The listing builds one solid part. Answer for the finished solid, in the listing's coordinates (mm). Face numbers are marked on the shaded views. Coordinates: 2 decimals unless noted, no trailing zeros. Loops run counter-clockwise (first coordinate to the right, second up) from the corner with the lowest first, then second, coordinate; pieces in that order, holes last. Notation, with made-up numbers: (5.5, 69.25) - (49.5, 69.25) arc R31 cw to (49.5, 94.25) - close; hole circle Ø8 at (22, 75.5). An arc over 180 degrees is marked (long way). Return JSON: item names as keys, results as strings. Group by question number.
1. Find the intervals of material crossed by line 1 along Y through (x, z) = (-659, -26.5); line 2 along Z through (x, y) = (303, -25.5); line 3 along Y through (x, z) = (-321.5, 32), in increasing order.
2. The mould has two halves that part along Z. Classify the marked faces 1, 2 and 3: pulls with the +Z half, pulls with the -Z half, needs draft (parallel to the pull), parting line crosses it, or undercut.
3. Section C-C (y = -14) is taken. Write down the section's boundary in (x, z).
4. Section B-B (z = 17.5) is taken. Write down the section's boundary in (x, y), and give its area (3 significant figures).
5. Section A-A (x = -591) is taken. Write down the section's boundary in (y, z), and give its area (3 significant figures).
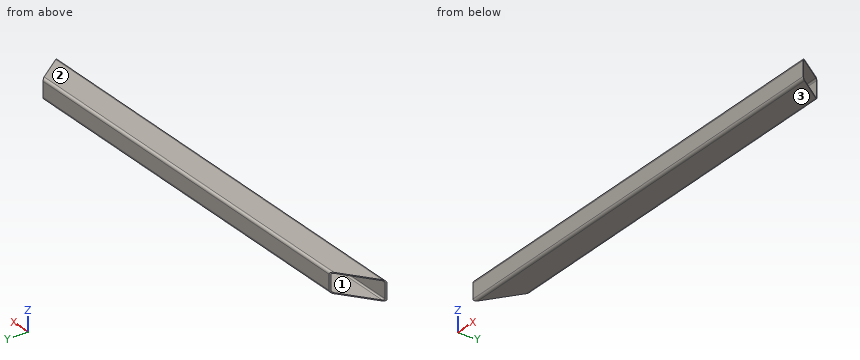
```python
from build123d import *

# Parameters (mm, degrees)
EL_MENT_M_CANO_SOUD_1_DEPTH = 1883.6164
EXTRUSION1_DEPTH            = 81
EXTRUSION2_DEPTH            = 81


with BuildPart() as part:
    # Esquisse15 → Elément mécano-soudé1 (new body)
    with BuildSketch(Plane.YZ.offset(-941.8082)):
        with BuildLine():
            Line((-50, 40), (50, 40))
            ThreePointArc((50, 40), (57.071067812, 37.071067812), (60, 30))
            Line((60, 30), (60, -30))
            ThreePointArc((60, -30), (57.071067812, -37.071067812), (50, -40))
            Line((50, -40), (-50, -40))
            ThreePointArc((-50, -40), (-57.071067812, -37.071067812), (-60, -30))
            Line((-60, -30), (-60, 30))
            ThreePointArc((-60, 30), (-57.071067812, 37.071067812), (-50, 40))
        make_face()
        with BuildLine():
            Line((-50, 36), (50, 36))
            ThreePointArc((50, 36), (54.242640687, 34.242640687), (56, 30))
            Line((56, 30), (56, -30))
            ThreePointArc((56, -30), (54.242640687, -34.242640687), (50, -36))
            Line((50, -36), (-50, -36))
            ThreePointArc((-50, -36), (-54.242640687, -34.242640687), (-56, -30))
            Line((-56, -30), (-56, 30))
            ThreePointArc((-56, 30), (-54.242640687, 34.242640687), (-50, 36))
        make_face(mode=Mode.SUBTRACT)
    extrude(amount=EL_MENT_M_CANO_SOUD_1_DEPTH)

    # Esquisse12 → Extrusion1 (cut, through all)
    with BuildSketch(Plane.XY.offset(40)):
        Polygon((941.8082, -60), (851.381713988, 60), (941.8082, 60), align=None)
        Polygon((-941.8082, -60), (-782.562821406, 60), (-941.8082, 60), align=None)
    extrude(amount=-EXTRUSION1_DEPTH, mode=Mode.SUBTRACT)

    # Esquisse13 → Extrusion2 (cut, through all)
    with BuildSketch(Plane.XY.offset(40)):
        Polygon((-1042.175315796, -60), (-925.191798589, -60), (-765.946419994, 60), (-882.929937201, 60), align=None)
    extrude(amount=-EXTRUSION2_DEPTH, mode=Mode.SUBTRACT)


solid = part.part
```
The answers:
{
 "1": {"line 1": "y = -60 to -56, 56 to 60", "line 2": "z = -40 to -36, 36 to 40", "line 3": "y = -59.8 to -55.66, 55.66 to 59.8"},
 "2": {"face 1": "undercut", "face 2": "pulls with the +Z half", "face 3": "pulls with the -Z half"},
 "3": {"outline": "(-864.15, -40) - (907.14, -40) - (907.14, -36) - (-864.15, -36) - close; (-864.15, 36) - (907.14, 36) - (907.14, 40) - (-864.15, 40) - close"},
 "4": {"outline": "(-925.19, -60) - (941.81, -60) - (938.79, -56) - (-919.88, -56) - close; (-771.25, 56) - (854.4, 56) - (851.38, 60) - (-765.95, 60) - close", "area": "13,900 mm2"},
 "5": {"outline": "(-60, -30) arc R10 ccw to (-50, -40) - (50, -40) arc R10 ccw to (60, -30) - (60, 30) arc R10 ccw to (50, 40) - (-50, 40) arc R10 ccw to (-60, 30) - close; hole (-56, -30) arc R6 ccw to (-50, -36) - (50, -36) arc R6 ccw to (56, -30) - (56, 30) arc R6 ccw to (50, 36) - (-50, 36) arc R6 ccw to (-56, 30) - close", "area": "1,480 mm2"}
}
